Input: dimensioned drawing with shaded views. Units: mm. Origin: part minimum x, y, z. Round coordinates to 2 decimals unless told otherwise and drop trailing zeros. Order: outer loops, then holes, each group sorted by start corner. A loop starts at its lowest first (then second) coordinate and runs counter-clockwise, first axis right, second up. Notation, with made-up numbers: M 66,-27 L 99,-27 A18 cw 99,-6 Z; hole C 48.5,66.25 d4. An arc over 180 degrees is marked long. Put each result on its own line as item: value. Start each with the question number.
1) Material intervals for probe 1 along Y at (x, z) = (42.5, 9); probe 2 along Z at (x, y) = (39, 68.5); probe 3 along Y at (x, z) = (75.5, 18.75), sorted ascending. Write a range as [from, to].
2) First-contact query: P1, Ø1, axis at x = 65, y = 54, coming from the -Z side; P2, Ø12, axis at y = 16.5, z = 3.5, coming from the -X side; P3, Ø12, axis at y = 56.5, z = 4, coming from the -X side; P4, Ø12, axis at x = 24, y = 75.5, coming from the +Z side. Flat tips, straight axial feed; report the tip coordinate or a pass-through.
3) Section A-A, the plane x = 42.5. Return loops of the section in (y, z), then the cut area to 3 significant figures.
4) Draft query along X for the marked faces 1 and 2. Return one class per face: pulls with the +X half, pulls with the -X half, needs draft (parallel to the pull), parting line crosses it, or undercut.
5) Section C-C, the plane z = 7.5. Return loops of the section in (x, y).
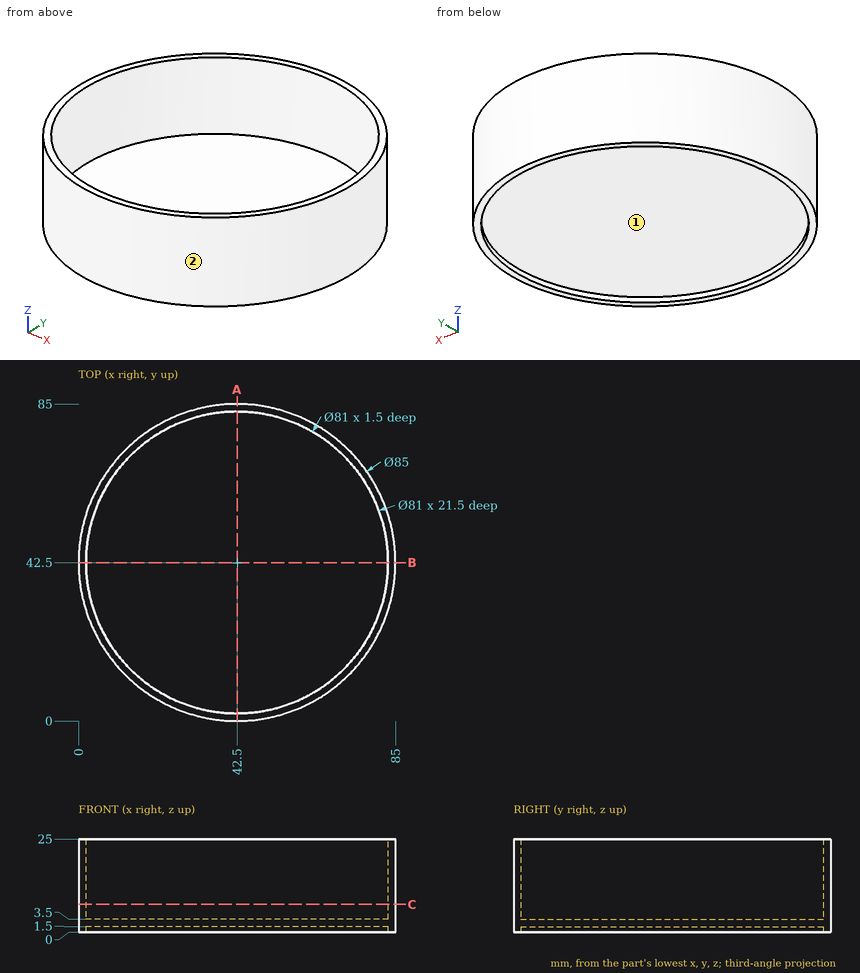
Result sheet:
1. probe 1: y = [0, 2], [83, 85]
1. probe 2: z = [1.5, 3.5]
1. probe 3: y = [15.72, 19.02], [65.98, 69.28]
2. P1: stops at z = 1.5
2. P2: stops at x = 5
2. P3: stops at x = 0.76
2. P4: stops at z = 25
3. outline: M 0,0 L 2,0 L 2,1.5 L 83,1.5 L 83,0 L 85,0 L 85,25 L 83,25 L 83,3.5 L 2,3.5 L 2,25 L 0,25 Z
3. area: 262 mm2
4. face 1: undercut
4. face 2: parting line crosses it
5. outline: C 42.5,42.5 d85; hole C 42.5,42.5 d81
